```python
from build123d import *

# Parameters (mm, degrees)
SKETCH1_W                 = 152.4
SKETCH1_H                 = 152.4
BOSS_EXTRUDE2_DEPTH       = 12
SKETCH2_W                 = 9.652
SKETCH2_H                 = 9.652
BOSS_EXTRUDE3_DEPTH       = 38.1
SKETCH3_W                 = 5.08
SKETCH3_H                 = 3.048
BOSS_EXTRUDE4_DEPTH       = 127
CHAMFER1_SIZE             = 0.508
CHAMFER1_SIZE2            = 0.03552282
CHAMFER2_SIZE             = 0.508
CHAMFER2_SIZE2            = 0.03552282
SKETCH4_W                 = 5.334
SKETCH4_H                 = 3.175
CUT_EXTRUDE3_DEPTH        = 149.86
SKETCH5_R                 = 4.445
BOSS_EXTRUDE5_DEPTH       = 15
F_2_0MM_DOWEL_HOLE1_D     = 2
F_2_0MM_DOWEL_HOLE1_DEPTH = 4.572
F_2_0MM_DOWEL_HOLE1_TIP   = 0.600860619
SHELL1_START              = 1.778
SHELL1_OUTLINE_W          = 148.844
SHELL1_OUTLINE_H          = 143.51
SHELL1_DEPTH              = 8.444
SHELL1_START_2            = 10.222
SHELL1_2_OUTLINE_W        = 6.096
SHELL1_2_OUTLINE_H        = 6.096
SHELL1_2_DEPTH            = 39.878
SHELL1_3_OUTLINE_W        = 148.844
SHELL1_3_OUTLINE_H        = 5.334
SHELL1_3_DEPTH            = 0.8565
SHELL1_START_3            = 9.3655
SHELL1_4_OUTLINE_W        = 148.844
SHELL1_4_OUTLINE_H        = 5.334
SHELL1_4_DEPTH            = 0.8565
SHELL1_START_4            = -7.752865101
SHELL1_5_OUTLINE_R        = 2.667
SHELL1_5_DEPTH            = 9.530865101
FILLET1_R                 = 1.27


with BuildPart() as part:
    # Sketch1 → Boss-Extrude2 (new body)
    with BuildSketch(Plane(origin=(0, 0, 0), x_dir=(1, 0, 0), z_dir=(0, 1, 0))):
        with Locations((53.878787879, -60.325)):
            Rectangle(SKETCH1_W, SKETCH1_H)
    extrude(amount=BOSS_EXTRUDE2_DEPTH)

    # Sketch2 → Boss-Extrude3 (add)
    with BuildSketch(Plane(origin=(0, 12, 0), x_dir=(1, 0, 0), z_dir=(0, 1, 0))):
        with Locations((-17.495212121, -131.699)):
            Rectangle(SKETCH2_W, SKETCH2_H)
    extrude(amount=BOSS_EXTRUDE3_DEPTH)

    # Sketch3 → Boss-Extrude4 (add)
    with BuildSketch(Plane.XY.offset(136.525)):
        with Locations((132.618787879, 6)):
            Rectangle(SKETCH3_W, SKETCH3_H)
    extrude(amount=-BOSS_EXTRUDE4_DEPTH)

    # Chamfer1
    chamfer1_edges = [part.edges().sort_by_distance(p)[0] for p in [
        (135.158787879, 7.524, 73.025),
    ]]
    chamfer1_side = [part.faces().sort_by_distance(p)[0] for p in [
        (132.618787879, 7.524, 73.025),
    ]]
    chamfer(chamfer1_edges, length=CHAMFER1_SIZE, length2=CHAMFER1_SIZE2, reference=chamfer1_side[0])

    # Chamfer2
    chamfer2_edges = [part.edges().sort_by_distance(p)[0] for p in [
        (135.158787879, 4.476, 73.025),
    ]]
    chamfer2_side = [part.faces().sort_by_distance(p)[0] for p in [
        (132.618787879, 4.476, 73.025),
    ]]
    chamfer(chamfer2_edges, length=CHAMFER2_SIZE, length2=CHAMFER2_SIZE2, reference=chamfer2_side[0])

    # Sketch4 → Cut-Extrude3 (cut)
    with BuildSketch(Plane.ZY.offset(22.321212121)):
        with Locations((-13.208, 6)):
            Rectangle(SKETCH4_W, SKETCH4_H)
    extrude(amount=-CUT_EXTRUDE3_DEPTH, mode=Mode.SUBTRACT)

    # Sketch5 → Boss-Extrude5 (add)
    with BuildSketch(Plane(origin=(0, 0, 0), x_dir=(1, 0, 0), z_dir=(0, 1, 0))):
        with Locations(Location((100.106787879, -9.125, 0), (0, 0, 270))):
            Circle(SKETCH5_R)
    extrude(amount=-BOSS_EXTRUDE5_DEPTH)

    # Ø2.0mm Dowel Hole1
    with Locations(Plane(origin=(0, -15, 0), x_dir=(-1, 0, 0), z_dir=(0, -1, 0))):
        with Locations((-100.106787879, -9.125)):
            Hole(F_2_0MM_DOWEL_HOLE1_D / 2, depth=F_2_0MM_DOWEL_HOLE1_DEPTH)
            with Locations((0, 0, -(F_2_0MM_DOWEL_HOLE1_DEPTH + F_2_0MM_DOWEL_HOLE1_TIP / 2))):  # 118° drill point
                Cone(0, F_2_0MM_DOWEL_HOLE1_D / 2, F_2_0MM_DOWEL_HOLE1_TIP, mode=Mode.SUBTRACT)

    # Shell1: read off the stored shape, not the designer's step
    # Shell1 outline → Shell1 (cut)
    with BuildSketch(Plane(origin=(0, 0, 0), x_dir=(1, 0, 0), z_dir=(0, 1, 0)).offset(SHELL1_START)):
        with Locations((53.878787879, -62.992)):
            Rectangle(SHELL1_OUTLINE_W, SHELL1_OUTLINE_H)
    extrude(amount=SHELL1_DEPTH, mode=Mode.SUBTRACT)

    # Shell1 2 outline → Shell1 2 (cut)
    with BuildSketch(Plane(origin=(0, 0, 0), x_dir=(1, 0, 0), z_dir=(0, 1, 0)).offset(SHELL1_START_2)):
        with Locations((-17.495212121, -131.699)):
            Rectangle(SHELL1_2_OUTLINE_W, SHELL1_2_OUTLINE_H)
    extrude(amount=SHELL1_2_DEPTH, mode=Mode.SUBTRACT)

    # Shell1 3 outline → Shell1 3 (cut)
    with BuildSketch(Plane(origin=(0, 0, 0), x_dir=(1, 0, 0), z_dir=(0, 1, 0)).offset(SHELL1_START)):
        with Locations((53.878787879, 11.43)):
            Rectangle(SHELL1_3_OUTLINE_W, SHELL1_3_OUTLINE_H)
    extrude(amount=SHELL1_3_DEPTH, mode=Mode.SUBTRACT)

    # Shell1 4 outline → Shell1 4 (cut)
    with BuildSketch(Plane(origin=(0, 0, 0), x_dir=(1, 0, 0), z_dir=(0, 1, 0)).offset(SHELL1_START_3)):
        with Locations((53.878787879, 11.43)):
            Rectangle(SHELL1_4_OUTLINE_W, SHELL1_4_OUTLINE_H)
    extrude(amount=SHELL1_4_DEPTH, mode=Mode.SUBTRACT)

    # Shell1 5 outline → Shell1 5 (cut)
    with BuildSketch(Plane(origin=(0, 0, 0), x_dir=(1, 0, 0), z_dir=(0, 1, 0)).offset(SHELL1_START_4)):
        with Locations((100.106787879, -9.125)):
            Circle(SHELL1_5_OUTLINE_R)
    extrude(amount=SHELL1_5_DEPTH, mode=Mode.SUBTRACT)

    # Shell1 6 outline → Shell1 6 (revolve, cut)
    with BuildSketch(Plane(origin=(100.106787879, 0, 9.125), x_dir=(1, 0, 0), z_dir=(0, 0, 1))):
        Polygon((0, -7.752865201), (2.667, -9.355360472), (2.667, -7.752865101), align=None)
    revolve(axis=Axis((100.106787879, 0, 9.125), (0, 1, 0)), mode=Mode.SUBTRACT)

    # Fillet1
    fillet1_edges = [part.edges().sort_by_distance(p)[0] for p in [
        (-22.321212121, 50.1, 131.699),
        (-17.495212121, 50.1, 136.525),
        (-12.669212121, 50.1, 131.699),
        (-17.495212121, 50.1, 126.873),
    ]]
    fillet(fillet1_edges, radius=FILLET1_R)


solid = part.part
```
The model under review builds one solid part; all positions refer to its coordinate system, in mm. A direction names the side the tool comes from. Round coordinates to 2 decimals unless told otherwise and drop trailing zeros. Loops run counter-clockwise (first coordinate to the right, second up) from the corner with the lowest first, then second, coordinate; pieces in that order, holes last. Notation, with made-up numbers: (-9.5, -25) -> (48.5, -25) arc R30 ccw to (48.5, 5) -> close; hole circle Ø10 at (11.5, -25.5). An arc over 180 degrees is marked (long way). Answer as a JSON object with one key per item and string values. Group by question number.
1) We need section A-A on x = 7. Write out the cut boundary in (y, z) (1 decimal).
2) We need section D-D on z = 67. Write out the cut boundary in (x, y).
3) For faces 5 (the face through (53, 1.778, 59)), 6 (the face through (52, 4.412, -13)), 7 (the face through (-18, 30, 128.651)), list the 3-axis set-ups (+Z, -Z, +X, -X, +Y, -Y) from which the entire face can be reached by the end or side of a thin tool; tool diameter is ignored.
4) For line 1 (Y direction, x = -12, z = 5); line 2 (Z direction, x = 13, y = 3) (3 decimals); line 3 (X direction, y = 2.5, z = 9), list the stretches that pass through material, from the lowest coordinate up. Write a range as [from, to].
5) For pin 1 Ø2 at (x, z) = (76.5, 105) entering from +Y; pin 2 Ø3.5 at (x, y) = (133, 5.5) entering from -Z (3 decimals); pin 3 Ø14.5 at (x, y) = (27, 24.5) entering from -Z; pin 4 Ø1 at (y, z) = (5, -13) entering from -X, all flat-tipped, find the tip position at first contact; note any pin that passes through.
6) Mouldability with a two-part tool opening along X and no side actions: class faces 1 (the face through (132, 7.524, 74)), 2 (the face through (-22.321, 11.6, 72)), 3 (the face through (-12.669, 30, 132)), 4 (the face through (-20.543, 10, 72)) as released by +X, released by -X, zero draft, split by the parting line, or undercut.
7) We need section C-C on y = 30. Write out the cut boundary in (x, z) (3 decimals).
8) We need section B-B on z = -5. Write out the cut boundary in (x, y), then the cut area to 3 significant figures.
Result set:
{
 "1": {"outline": "(0, -15.9) -> (4.4, -15.9) -> (4.4, -10.5) -> (7.6, -10.5) -> (7.6, -15.9) -> (12, -15.9) -> (12, 136.5) -> (0, 136.5) -> close; hole (1.8, -14.1) -> (2.6, -14.1) -> (2.6, -8.8) -> (9.4, -8.8) -> (9.4, -14.1) -> (10.2, -14.1) -> (10.2, 134.7) -> (1.8, 134.7) -> close"},
 "2": {"outline": "(-22.32, 0) -> (130.08, 0) -> (130.08, 4.48) -> (134.65, 4.48) -> (135.16, 4.51) -> (135.16, 7.49) -> (134.65, 7.52) -> (130.08, 7.52) -> (130.08, 12) -> (-22.32, 12) -> close; hole (-20.54, 1.78) -> (128.3, 1.78) -> (128.3, 10.22) -> (-20.54, 10.22) -> close"},
 "3": {"face 5": "none", "face 6": "-Z, -X", "face 7": "+Y"},
 "4": {"line 1": "[0, 1.78], [10.22, 12]", "line 2": "[-15.875, -8.763], [134.747, 136.525]", "line 3": "[-22.32, -20.54], [128.3, 130.08]"},
 "5": {"pin 1": "y = 12", "pin 2": "z = 9.525", "pin 3": "through", "pin 4": "x = 127.54"},
 "6": {"face 1": "zero draft", "face 2": "released by -X", "face 3": "released by +X", "face 4": "undercut"},
 "7": {"outline": "(-22.321, 126.873) -> (-12.669, 126.873) -> (-12.669, 136.525) -> (-22.321, 136.525) -> close; hole (-20.543, 128.651) -> (-14.447, 128.651) -> (-14.447, 134.747) -> (-20.543, 134.747) -> close"},
 "8": {"outline": "(-22.32, 0) -> (130.08, 0) -> (130.08, 12) -> (-22.32, 12) -> close; hole (-20.54, 1.78) -> (128.3, 1.78) -> (128.3, 10.22) -> (-20.54, 10.22) -> close", "area": "572 mm²"}
}
